Could you check a few things on this model? Use its own coordinates, in mm. A direction names the side the tool comes from. Round coordinates to 2 decimals unless told otherwise and drop trailing zeros. Loops run counter-clockwise (first coordinate to the right, second up) from the corner with the lowest first, then second, coordinate; pieces in that order, holes last. Notation, with made-up numbers: M 2,-3 L 14,-3 A13 ccw 14,14 Z; hole C -9.75,64 d5. An arc over 180 degrees is marked long. Answer in a Markdown table with one row per item.
Autodesk Inventor part; units mm, degrees
ref_plane "YZ Plane" through (0, 0, 0) normal (1, 0, 0) x (0, 1, 0)
ref_plane "XZ Plane" through (0, 0, 0) normal (0, 1, 0) x (-1, 0, 0)
ref_plane "XY Plane" through (0, 0, 0) normal (0, 0, 1) x (1, 0, 0)
sketch "Sketch1" plane through (0, 0, 0) normal (0, 0, 1) x (1, 0, 0)
  line L0 (-31, 6.1) -> (0, 6.1)
  line L1 (0, 6.1) -> (31, 6.1)
  line L2 (0, 10.5424) -> (0, 0) construction
  line L3 (31, 9.75) -> (31, 6.1)
  line L4 (77, 9.75) -> (77, 0)
  line L5 (46.4247, 9.75) -> (46.4247, 4.1503)
  line L6 (46.4247, 4.1503) -> (48.4247, 4.1503)
  line L7 (48.4247, 4.1503) -> (48.4247, 9.75)
  line L8 (31, 9.75) -> (46.4247, 9.75) construction
  line L9 (31, 9.75) -> (46.4247, 9.75)
  line L10 (62.7124, 9.75) -> (62.7124, 9.1289)
  line L11 (62.7124, 9.1289) -> (62.9117, 9.1289)
  line L12 (62.9117, 9.1289) -> (62.9117, 9.75)
  line L13 (48.4247, 9.75) -> (62.7124, 9.75) construction
  line L14 (62.9117, 9.75) -> (77, 9.75) construction
  line L15 (48.4247, 9.75) -> (62.7124, 9.75)
  line L16 (62.9117, 9.75) -> (77, 9.75)
  line L17 (-31, 8.1) -> (-60.2, 8.1)
  line L18 (-60.2, 8.1) -> (-60.2, 0)
  line L19 (-31, 8.1) -> (-31, 6.1)
  line L20 (-60.2, 4.875) -> (-63.45, 4.875)
  line L21 (-66.7, 0) -> (-60.2, 0)
  line L22 (-63.45, 4.875) -> (-63.45, 2.7274)
  line L23 (-63.45, 2.7274) -> (-65.075, 2.7274)
  line L24 (-65.075, 2.7274) -> (-65.075, 1.425)
  line L25 (-65.075, 1.425) -> (-66.7, 1.425)
  line L26 (-66.7, 1.425) -> (-66.7, 0)
  line L27 (-60.2, 0) -> (77, 0)
  line L28 (-95.44, 0) -> (105.74, 0)
  dimension "d1" = 31
  dimension "d2" = 31
  dimension "d3" = 6.1
  dimension "d4" = 46
  dimension "d6" = 2
  dimension "d7" = 29.2
  dimension "d8" = 8.1
  dimension "d10" = 1.425
  dimension "d11" = 6.5
revolve "Revolution1" add sketch "Sketch1" angle 360 about axis through (-10, 0, 0) along (1, 0, 0)
sketch "Sketch2" plane through (77, 0, 0) normal (1, 0, 0) x (0, 0, -1)
  circle A0 centre (0, 0) radius 9.75
extrude "Extrusion1" cut sketch "Sketch2" against normal up to surface (30.5753 mm away)
sketch "Sketch3" plane through (46.4247, 0, 0) normal (1, 0, 0) x (0, 0, -1)
  circle A0 centre (0, 0) radius 6.1
  dimension "d15" = 12.2
extrude "Extrusion2" add sketch "Sketch3" along normal blind 25
sketch "Sketch4" plane through (71.4247, 0, 0) normal (1, 0, 0) x (0, 0, -1)
  circle A0 centre (0, 0) radius 4.875
  circle A1 centre (0, 0) radius 6.1
  line L0 (0, 0) -> (0, 10.6003)
  line L1 (0, 0) -> (6.8931, 6.8955)
  circle A2 centre (0, 0) radius 9.75
  circle A3 centre (0, 0) radius 8.1
  circle A4 centre (0, 0) radius 9.75
extrude "Extrusion3" cut sketch "Sketch4" against normal blind 5 contours A0 L0 L1 | L1 L0 A0
properties part number "PH Monitor"
1) Which directions (+Z, -Z, +X, -X, +Y, -Y) give clear straight access to the entire face, cutting with the end or side of a thin tool? Please do faces 4 (the face through (-65.075, 1.2, -1.2)), 5 (the face through (46.425, -0.1, -6.4)), 6 (the face through (0.434, -6.094, 0.268)).
Computed:
| item | result |
|---|---|
| face 4 | -X |
| face 5 | +X |
| face 6 | none |
2) Will these pins go through, and if not, where does the flat tip stop? P1, Ø5, axis at x = -7, y = 7, coming from the +Z side; P2, Ø5, axis at y = -3.5, z = -0.5, coming from the +X side; P3, Ø5, axis at x = -16, y = 3, coming from the +Z side; P4, Ø1.5, axis at x = 55.5, z = 3, coming from the -Y side.
Computed:
| item | result |
|---|---|
| P1 | stops at z = 4.12 |
| P2 | stops at x = 71.42 |
| P3 | stops at z = 6.08 |
| P4 | stops at y = -5.67 |
3) I need wall thicknesses on line 1 (Y direction, x = 69.1, z = 0) (3 decimals); line 2 (X direction, y = 5.25, z = 4.25); line 3 (Y direction, x = 50, z = -0.5). Which ranges of each line are inside material? Lowest first, please.
Computed:
| item | result |
|---|---|
| line 1 | y = -6.1 to -4.875, 4.875 to 6.1 |
| line 2 | x = -60.2 to -31, 31 to 46.42 |
| line 3 | y = -6.08 to 6.08 |
4) I want a section at C-C, the plane x = 39.5. Please give me the cut outline in (y, z), plus the area to 3 significant figures.
Computed:
| item | result |
|---|---|
| outline | C 0,0 d19.5 |
| area | 299 mm² |
5) I want a section at D-D, the plane x = -54. Please give me the cut outline in (y, z).
Computed:
| item | result |
|---|---|
| outline | C 0,0 d16.2 |
6) If we mould it in two halves opening along X, with no side actions, what happens to faces 1 (the face through (-65.9, -1.13, 0.87)), 2 (the face through (-31, 2, 6)), 3 (the face through (-63.45, 2.1, -2.1))? For each: released by +X, released by -X, zero draft, split by the parting line, or undercut.
Computed:
| item | result |
|---|---|
| face 1 | zero draft |
| face 2 | undercut |
| face 3 | released by -X |
